Input: part model. Units: mm. Frame: model coordinates. Face numbers are marked on the shaded views. A direction names the side the tool comes from. Round coordinates to 2 decimals unless told otherwise and drop trailing zeros. Loops run counter-clockwise (first coordinate to the right, second up) from the corner with the lowest first, then second, coordinate; pieces in that order, holes last.
1) Draft query along X for the marked faces 1, 2 and 3. Return one class per face: pulls with the +X half, pulls with the -X half, needs draft (parallel to the pull), parting line crosses it, or undercut.
2) Ray query, line 1 along Y through (x, z) = (4, 10.5); line 2 along X through (y, z) = (-0.25, 26); line 3 along Y through (x, z) = (-6.5, 8.5). Return the intervals inside material, ascending.
3) Access query for the marked faces 4, 5 and 6. Directions: +Z, -Z, +X, -X, +Y, -Y. A direction counts if a zero-diameter tool reaches every point of the face in a straight line with its end or side. Return the directions, or none.
4) Section B-B, the plane x = 3. Return loops of the section in (y, z), and give its area (3 significant figures).
5) Section D-D, the plane z = 31.5. Return loops of the section in (x, y), and give its area (3 significant figures).
6) Section C-C, the plane y = 3.5. Return loops of the section in (x, z).
7) Section A-A, the plane y = -4.5. Return loops of the section in (x, z), and give its area (3 significant figures).
Autodesk Inventor part; units mm, degrees
ref_plane "YZ Plane" through (0, 0, 0) normal (1, 0, 0) x (0, 1, 0)
ref_plane "XZ Plane" through (0, 0, 0) normal (0, 1, 0) x (-1, 0, 0)
ref_plane "XY Plane" through (0, 0, 0) normal (0, 0, 1) x (1, 0, 0)
sketch "Sketch1" plane through (0, 0, 0) normal (0, 0, 1) x (1, 0, 0)
  line L0 (-12, 10.5) -> (12, 10.5)
  line L1 (12, 10.5) -> (12, -10.5)
  line L2 (12, -10.5) -> (-12, -10.5)
  line L3 (-12, -10.5) -> (-12, 10.5)
  point P0 (0, 0)
  dimension "d0" = 24
  dimension "d1" = 12
  dimension "d2" = 21
  dimension "d3" = 10.5
extrude "Blok" add sketch "Sketch1" along normal blind 33.5
sketch "Sketch2" plane through (12, -10.5, 0) normal (1, 0, 0) x (0, 0, -1)
  line L0 (0, 0) -> (-33.5, 0)
  line L1 (-28.5, 0) -> (-28.5, 21) construction
  line L2 (0, 21) -> (-33.5, 21)
  circle A0 centre (-10.5, 10.5) radius 7.5
  line L3 (0, 21) -> (0, 0)
  line L4 (-32.5, 21) -> (-32.5, 0) construction
  line L5 (-24.5, 21) -> (-24.5, 0) construction
  line L6 (0, 0) -> (-33.5, 0)
  line L7 (-33.5, 0) -> (-33.5, 21)
  point P0 (0, 10.5)
  dimension "d6" = 15
  dimension "d7" = 18
  dimension "d8" = 10.5
  dimension "d9" = 10.5
  dimension "d10" = 10.5
  dimension "d11" = 4
  dimension "d12" = 4
  dimension "d13" = 1
extrude "Lejehul" cut sketch "Sketch2" against normal up to surface (24 mm away) contours A0
sketch "Sketch3" plane through (-12, 10.5, 0) normal (0, 1, 0) x (1, 0, 0)
  line L0 (0, -18) -> (0, -3) construction
  line L1 (24, -3) -> (24, -18) construction
  line L2 (24, 0) -> (24, -33.5)
  line L3 (0, -18) -> (24, -18) construction
  line L4 (0, -3) -> (24, -3) construction
  line L5 (0, 0) -> (0, -33.5)
  line L6 (0, -3) -> (24, -18) construction
  line L7 (24, -10.5) -> (0, -10.5) construction
  line L8 (24, -28.5) -> (0, -28.5) construction
  arc A0 (18.2766, -30.7943) -> (11.7234, -30.7943) centre (15, -28.5) ccw
  line L9 (11.7234, -30.7943) -> (8.2936, -25.896) construction
  line L10 (18.2766, -30.7943) -> (20.9993, -26.9059) construction
  line L11 (11.7234, -30.7943) -> (18.2766, -30.7943) construction
  line L12 (11.7234, -30.7943) -> (9.8288, -33.5)
  line L13 (18.2766, -30.7943) -> (20.1712, -33.5)
  line L14 (9.8288, -33.5) -> (0, -33.5) construction
  line L15 (20.1712, -33.5) -> (24, -33.5) construction
  line L16 (24, -33.5) -> (24, -33.5)
  line L17 (0, -33.5) -> (0, -33.5)
  line L18 (0, 0) -> (24, 0)
  line L19 (24, -33.5) -> (0, -33.5) construction
  line L20 (9.8288, -33.5) -> (20.1712, -33.5)
  line L21 (15, -28.5) -> (15, -33.5)
  point P0 (12, 0)
  point P1 (12, -10.5)
  dimension "d19" = 18
  dimension "d20" = 8
  dimension "d24" = 110
  dimension "d25" = 110
  dimension "d29" = 9
  dimension "d30" = 35
extrude "Tværstang" cut sketch "Sketch3" against normal blind 18
sketch "Sketch4" plane through (12, -10.5, 0) normal (1, 0, 0) x (0, 0, -1)
  line L0 (-29.5, 7) -> (-26.5, 7)
  line L1 (-26.5, 7) -> (-26.5, 19)
  line L2 (-26.5, 19) -> (-29.5, 19)
  line L3 (-29.5, 19) -> (-29.5, 7)
  line L4 (0, 0) -> (-33.5, 0)
  line L5 (-33.5, 0) -> (-33.5, 21)
  line L6 (-24.5, 2) -> (-24.5, 9) construction
  line L7 (0, 21) -> (-33.5, 21)
  point P0 (0, 10.5)
  dimension "d32" = 3
  dimension "d34" = 4
  dimension "d35" = 2
  dimension "d37" = 2
  dimension "d41" = 12
revolve "Revolution1" cut sketch "Sketch4" angle 360 about axis through (12, -8.5, 24.5) along (0, 1, 0)
sketch "Sketch5" plane through (-12, -10.5, 0) normal (-1, 0, 0) x (0, 0, 1)
  line L0 (26.5, 7) -> (29.5, 7)
  line L1 (26.5, 19) -> (26.5, 7)
  line L2 (29.5, 19) -> (26.5, 19)
  line L3 (29.5, 7) -> (29.5, 19)
  line L4 (24.5, 19) -> (24.5, 12)
  point P0 (0, 10.5)
  dimension "d38" = 2
revolve "Revolution2" cut sketch "Sketch5" angle 360 about axis through (-12, 8.5, 24.5) along (0, -1, 0)
fillet "Fillet1" radius 1 8 edges at (7, -3.5, 24.5) (10, -3.5, 24.5) (7, 8.5, 24.5) (10, 8.5, 24.5) (-7, 8.5, 24.5) (-10, 8.5, 24.5) (-7, -3.5, 24.5) (-10, -3.5, 24.5)
equation "\"d8\" = d9"
equation "\"d12\" = d11"
equation "\"d25\" = d24"
properties part number "XY v2"
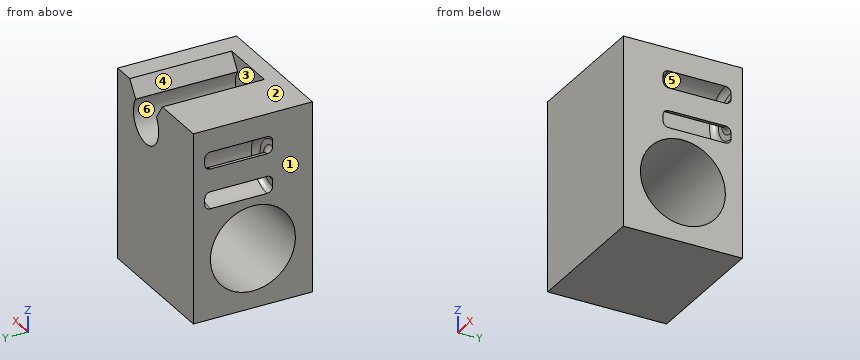
Final values:
1. face 1: pulls with the -X half
1. face 2: needs draft
1. face 3: undercut
2. line 1: y = -10.5 to -7.5, 7.5 to 10.5
2. line 2: x = -12 to -10.68, -7.23 to -0.12, 6.12 to 7.23, 10.68 to 12
2. line 3: y = -10.5 to -7.23, 7.23 to 10.5
3. face 4: +Z, +Y
3. face 5: none
3. face 6: +Y
4. outline: (-10.5, 0) - (10.5, 0) - (10.5, 24.5) - (-7.5, 24.5) - (-7.5, 33.5) - (-10.5, 33.5) - close; hole circle Ø15 at (0, 10.5)
4. area: 365 mm2
5. outline: (-12, -10.5) - (12, -10.5) - (12, 10.5) - (6.77, 10.5) - (6.77, -7.5) - (-0.77, -7.5) - (-0.77, 10.5) - (-12, 10.5) - close
5. area: 368 mm2
6. outline: (-12, 0) - (12, 0) - (12, 3.87) - (-12, 3.87) - close; (-12, 17.13) - (12, 17.13) - (12, 19.5) arc R5 cw to (12, 29.5) - (12, 33.5) - (8.17, 33.5) - (6.28, 30.79) arc R4 cw (long way) to (-0.28, 30.79) - (-2.17, 33.5) - (-12, 33.5) - (-12, 29.5) arc R5 cw to (-12, 19.5) - close; (-12, 22.5) arc R2 ccw to (-12, 26.5) - close; (12, 22.5) - (12, 26.5) arc R2 ccw to start
7. outline: (-12, 0) - (12, 0) - (12, 4.5) - (-12, 4.5) - close; (-12, 16.5) - (12, 16.5) - (12, 33.5) - (8.17, 33.5) - (6.28, 30.79) arc R4 cw (long way) to (-0.28, 30.79) - (-2.17, 33.5) - (-12, 33.5) - close
7. area: 451 mm2
